Geometry check sheet. Reference: drawing and pictorial views, mm from the part's lowest x, y, z. A direction names the side the tool comes from. Round coordinates to 2 decimals unless told otherwise and drop trailing zeros. Write each loop counter-clockwise with the first axis right and the second up, starting at its lowest first coordinate (ties: lowest second). Pieces come first, ordered by that corner, then holes.
Item 1: Section check A-A, the plane z = 47. Record the cut outline in (x, y) (1 decimal), plus the area to 3 significant figures.
Item 2: Section check C-C, the plane x = 47.5. Record the cut outline in (y, z) (1 decimal), plus the area to 3 significant figures.
Item 3: Set-up check for the marked faces 1 and 2: record each of +Z, -Z, +X, -X, +Y, -Y from which the full face is reachable in a straight line by a thin tool's end or side.
Item 4: Material ranges on line 1 along Z through (x, y) = (50, 95) (1 decimal); line 2 along X through (y, z) = (41.5, 46.5) (1 decimal), recorded low to high.
Item 5: Section check B-B, the plane y = 45. Record the cut outline in (x, z) (1 decimal), plus the area to 3 significant figures.
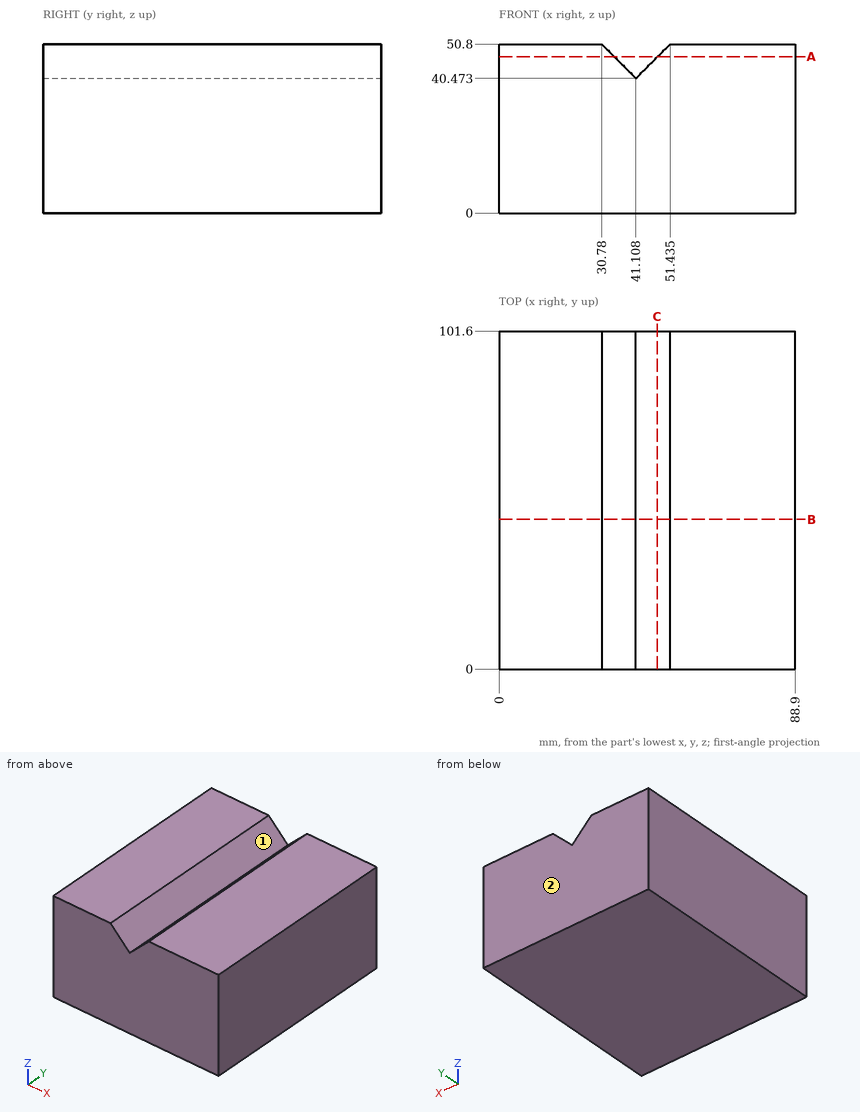
Values found:
1. outline: (0, 0) - (34.6, 0) - (34.6, 101.6) - (0, 101.6) - close; (47.6, 0) - (88.9, 0) - (88.9, 101.6) - (47.6, 101.6) - close
1. area: 7,710 mm2
2. outline: (0, 0) - (101.6, 0) - (101.6, 46.9) - (0, 46.9) - close
2. area: 4,760 mm2
3. face 1: +Z, +Y, -Y
3. face 2: +Z, -Z, +X, -X, +Y
4. line 1: z = 0 to 49.4
4. line 2: x = 0 to 35.1, 47.1 to 88.9
5. outline: (0, 0) - (88.9, 0) - (88.9, 50.8) - (51.4, 50.8) - (41.1, 40.5) - (30.8, 50.8) - (0, 50.8) - close
5. area: 4,410 mm2
